Read the model definition and answer for the solid it produces. Units are mm, in the model's axes. Face numbers are marked on the shaded views. A direction names the side the tool comes from. Coordinates: 2 decimals unless noted, no trailing zeros. Order: outer loops, then holes, each group sorted by start corner. A loop starts at its lowest first (then second) coordinate and runs counter-clockwise, first axis right, second up. Notation, with made-up numbers: (-17.5, -31.75) -> (13.5, -31.75) arc R19 cw to (13.5, -2.75) -> close; hole circle Ø1 at (61.5, 53.5). An arc over 180 degrees is marked (long way). Answer in a Markdown table with one row per item.
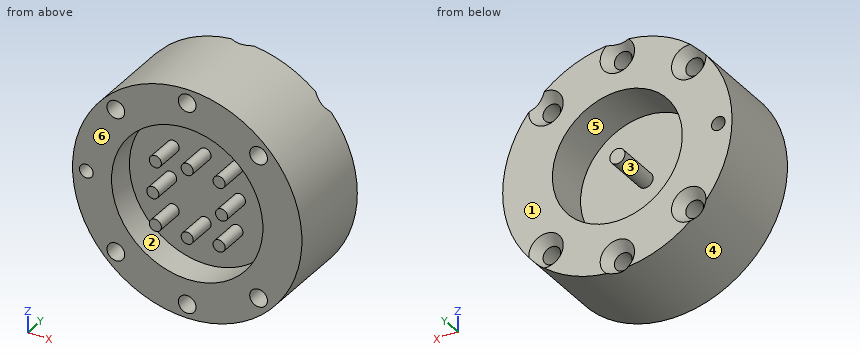
from build123d import *

# Parameters (mm, degrees)
OUTER_R                                        = 19.05
BODY_DEPTH                                     = 14.986
INNER_R                                        = 12.573
POCKET_DEPTH                                   = 4.826
CSK_FOR_4_FLAT_HEAD_MACHINE_SCREW1_D           = 2.9464
CSK_FOR_4_FLAT_HEAD_MACHINE_SCREW1_CSINK_D     = 5.715
CSK_FOR_4_FLAT_HEAD_MACHINE_SCREW1_CSINK_ANGLE = 82
SCREW_HOLES_COUNT                              = 4
POST_START                                     = 4.826
POST_SKETCH_R                                  = 1.0033
POST_DEPTH                                     = 4.826
POSTS_COUNT                                    = 4
CUT_EXTRUDE1_START                             = 14.986
SOLONOID_SKETCH_R                              = 10.795
SOLONOID_SKETCH_R_2                            = 1.2573
CUT_EXTRUDE1_DEPTH                             = 7.62
F_4_40_TAPPED_HOLE1_D                          = 2.2606


with BuildPart() as part:
    # outer → Body (new body)
    with BuildSketch(Plane(origin=(0, 0, 0), x_dir=(1, 0, 0), z_dir=(0, 1, 0))):
        with Locations(Location((0, 0, 0), (0, 0, 90))):
            Circle(OUTER_R)
    extrude(amount=BODY_DEPTH)

    # inner → Pocket (cut)
    with BuildSketch(Plane(origin=(0, 0, 0), x_dir=(1, 0, 0), z_dir=(0, 1, 0))):
        with Locations(Location((0, 0, 0), (0, 0, 270))):
            Circle(INNER_R)
    extrude(amount=POCKET_DEPTH, mode=Mode.SUBTRACT)

    # CSK for #4 Flat Head Machine Screw1 (through all)
    with Locations(Plane(origin=(0, 14.986, 0), x_dir=(1, 0, 0), z_dir=(0, 1, 0))):
        with Locations((-11.85393808, 11.85393808)):
            csk_for_4_flat_head_machine_screw1 = CounterSinkHole(CSK_FOR_4_FLAT_HEAD_MACHINE_SCREW1_D / 2, CSK_FOR_4_FLAT_HEAD_MACHINE_SCREW1_CSINK_D / 2, counter_sink_angle=CSK_FOR_4_FLAT_HEAD_MACHINE_SCREW1_CSINK_ANGLE)

    # Screw Holes: CSK for #4 Flat Head Machine Screw1 ×4 about axis
    screw_holes_axis = Axis((0, 0, 0), (0, 1, 0))
    for i in range(1, SCREW_HOLES_COUNT):
        add(csk_for_4_flat_head_machine_screw1.rotate(screw_holes_axis, i * 360 / SCREW_HOLES_COUNT), mode=Mode.SUBTRACT)

    # Post Sketch → Post (add)
    with BuildSketch(Plane(origin=(0, 0, 0), x_dir=(1, 0, 0), z_dir=(0, 1, 0)).offset(POST_START)):
        with Locations(Location((0, -5.715, 0), (0, 0, 270))):
            Circle(POST_SKETCH_R)
        with Locations(Location((5.298351111, -5.298351111, 0), (0, 0, 270))):
            Circle(POST_SKETCH_R)
    post = extrude(amount=-POST_DEPTH)

    # Posts: Post ×4 about axis
    posts_axis = Axis((0, 0, 0), (0, 1, 0))
    for i in range(1, POSTS_COUNT):
        add(post.rotate(posts_axis, i * 360 / POSTS_COUNT))

    # Solonoid Sketch → Cut-Extrude1 (cut)
    with BuildSketch(Plane(origin=(0, 0, 0), x_dir=(1, 0, 0), z_dir=(0, 1, 0)).offset(CUT_EXTRUDE1_START)):
        with Locations(Location((0, 0, 0), (0, 0, 270))):
            Circle(SOLONOID_SKETCH_R)
        with Locations(Location((0, 0, 0), (0, 0, 270))):
            Circle(SOLONOID_SKETCH_R_2, mode=Mode.SUBTRACT)
    extrude(amount=-CUT_EXTRUDE1_DEPTH, mode=Mode.SUBTRACT)

    # Sketch-Pattern1: CSK for #4 Flat Head Machine Screw1 at 2 more places
    with Locations((11.853938, 0, -4.910062), (11.853938, 0, 28.617938)):
        add(csk_for_4_flat_head_machine_screw1, mode=Mode.SUBTRACT)

    # #4-40 Tapped Hole1 (through all)
    with Locations(Plane(origin=(0, 14.986, 0), x_dir=(1, 0, 0), z_dir=(0, 1, 0))):
        with Locations((-16.764, 0)):
            Hole(F_4_40_TAPPED_HOLE1_D / 2)


solid = part.part
Q1. The part is cut by section B-B (y = 3.5). Give the number of separate pieces and of enclosed holes in the cut face, then the cut area to 3 significant figures.
Outcome:
| item | result |
|---|---|
| separate pieces | 9 |
| enclosed holes | 8 |
| area | 624 mm² |
Q2. Consider line 1 (Z direction, x = -1, y = 10.5); line 2 (X direction, y = 3, z = -5); line 3 (Z direction, x = 13, y = 1.75). Determine where each line is inside the solid, lowest interval first.
Outcome:
| item | result |
|---|---|
| line 1 | -19.02 to -17.85, -15.68 to -10.75, -0.76 to 0.76, 10.75 to 15.68, 17.85 to 19.02 |
| line 2 | -18.38 to -11.54, -6.26 to -4.34, -0.7 to 0.7, 4.34 to 6.26, 11.54 to 18.38 |
| line 3 | -13.92 to -12.78, -10.93 to 10.93, 12.78 to 13.92 |
Q3. Given pin 1 (1 mm diameter, centred on y = 1.5, z = 2.5, fed in from -X); pin 2 (3 mm diameter, centred on x = -8.5, y = 1.5, fed in from -Z); pin 3 (8 mm diameter, centred on x = 7.5, y = 2.5, fed in from -Z), each flat-ended and moving along its own axis, determine where each tip first touches the part or whether it passes through.
Outcome:
| item | result |
|---|---|
| pin 1 | x = -18.94 |
| pin 2 | z = -17.72 |
| pin 3 | z = -18.73 |
Q4. For the marked faces 1, 2 and 3, determine the directions among +Z, -Z, +X, -X, +Y, -Y from which every point of the face is accessible in a straight line to the end or side of a thin tool.
Outcome:
| item | result |
|---|---|
| face 1 | +Z, -Z, +X, -X, +Y |
| face 2 | -Y |
| face 3 | +Y |
Q5. The part is cut by section A-A (z = 0). Write down the section's boundary in (x, y) (3 decimals), then the cut area to 3 significant figures.
Outcome:
| item | result |
|---|---|
| outline | (-19.05, 0) -> (-17.894, 0) -> (-17.894, 14.986) -> (-19.05, 14.986) -> close; (-15.634, 0) -> (-12.573, 0) -> (-12.573, 4.826) -> (-6.718, 4.826) -> (-6.718, 0) -> (-4.712, 0) -> (-4.712, 4.826) -> (4.712, 4.826) -> (4.712, 0) -> (6.718, 0) -> (6.718, 4.826) -> (12.573, 4.826) -> (12.573, 0) -> (19.05, 0) -> (19.05, 14.986) -> (10.795, 14.986) -> (10.795, 7.366) -> (1.257, 7.366) -> (1.257, 14.986) -> (-1.257, 14.986) -> (-1.257, 7.366) -> (-10.795, 7.366) -> (-10.795, 14.986) -> (-15.634, 14.986) -> close |
| area | 290 mm² |
Q6. For a pull along Z with two mould halves and no side action, classify the marked faces 4, 5 and 6 as pulls with the +Z half, pulls with the -Z half, needs draft (parallel to the pull), parting line crosses it, or undercut.
Outcome:
| item | result |
|---|---|
| face 4 | parting line crosses it |
| face 5 | undercut |
| face 6 | needs draft |
